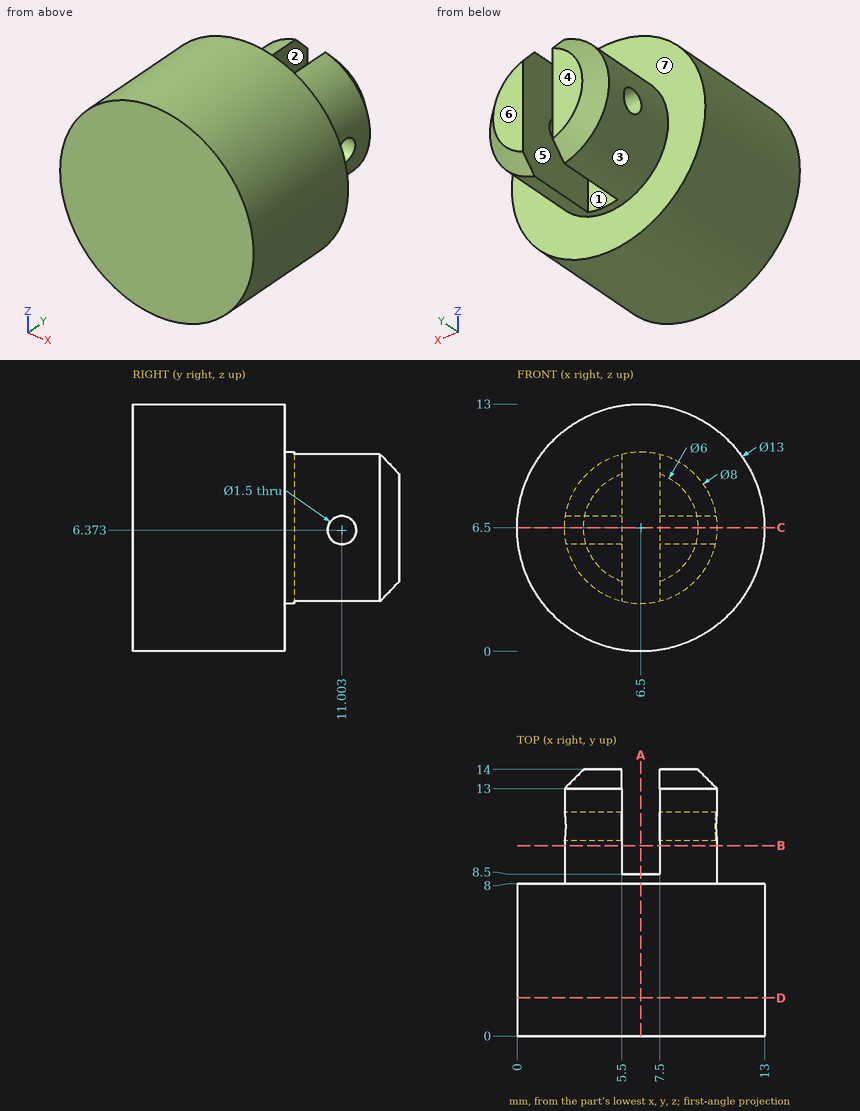
Here's the drawing with two shaded views (mm, measured from the low corner). I have some questions. A direction names the side the tool comes from. Round coordinates to 2 decimals unless told otherwise and drop trailing zeros. Order: outer loops, then holes, each group sorted by start corner. A loop starts at its lowest first (then second) coordinate and runs counter-clockwise, first axis right, second up. Notation, with made-up numbers: (86, 76.25) -> (100, 76.25) arc R17 cw to (100, 97.25) -> close; hole circle Ø5 at (68.25, 38.5). An arc over 180 degrees is marked (long way). Use a Markdown table: item, result. Add a question column.
(1) If we mould it in two halves opening along X, with no side actions, what happens to the marked faces 1, 2, 3 and 4? For each: released by +X, released by -X, zero draft, split by the parting line, or undercut.
(2) Suppose I cut it at D-D, the plane y = 2. Please give me the cut outline in (x, z).
(3) For pin 1 Ø1.2 at (y, z) = (11, 6.37) entering from -X; pin 2 Ø1.7 at (y, z) = (11, 6.37) entering from -X; pin 3 Ø4.5 at (y, z) = (10.5, 7) entering from +X; pin 4 Ø4 at (x, z) = (10.5, 3) entering from +Y (1 decimal), each with a flat end and sliding along its axis, tell me the tip position at first contact or that it passes through.
(4) Suppose I cut it at A-A, the plane x = 6.5. Please give me the cut outline in (y, z), and give its area (3 significant figures).
(5) Suppose I cut it at C-C, the plane z = 6.5. Please give me the cut outline in (x, y), and give its area (3 significant figures).
(6) Suppose I cut it at B-B, the plane y = 10. Please give me the cut outline in (x, z).
(7) I need wall thicknesses on line 1 along Y through (x, z) = (9.5, 12); line 2 along Y through (x, z) = (3.25, 7) (1 decimal); line 3 along X through (y, z) = (11, 9.75). Which ranges of each line are inside material? Lowest first, please.
(8) For the marked faces 5, 6 and 7, which set-ups out of +Z, -Z, +X, -X, +Y, -Y let a thin tool reach every point of the face, with its end or its side?
Verdict:
| question | item | result |
|---|---|---|
| 1 | face 1 | undercut |
| 1 | face 2 | undercut |
| 1 | face 3 | split by the parting line |
| 1 | face 4 | zero draft |
| 2 | outline | circle Ø13 at (6.5, 6.5) |
| 3 | pin 1 | through |
| 3 | pin 2 | x = 2.5 |
| 3 | pin 3 | x = 10.5 |
| 3 | pin 4 | y = 13.7 |
| 4 | outline | (0, 0) -> (8, 0) -> (8, 2.5) -> (8.5, 2.5) -> (8.5, 10.5) -> (8, 10.5) -> (8, 13) -> (0, 13) -> close |
| 4 | area | 108 mm2 |
| 5 | outline | (0, 0) -> (13, 0) -> (13, 8) -> (10.5, 8) -> (10.5, 10.26) -> (7.5, 10.26) -> (7.5, 8.5) -> (5.5, 8.5) -> (5.5, 10.26) -> (2.5, 10.26) -> (2.5, 8) -> (0, 8) -> close; (2.5, 11.74) -> (5.5, 11.74) -> (5.5, 14) -> (3.5, 14) -> (2.5, 13) -> close; (7.5, 11.74) -> (10.5, 11.74) -> (10.5, 13) -> (9.5, 14) -> (7.5, 14) -> close |
| 5 | area | 131 mm2 |
| 6 | outline | (5.5, 2.63) -> (5.5, 10.37) arc R4 ccw to start; (7.5, 2.63) arc R4 ccw to (7.5, 10.37) -> close |
| 7 | line 1 | 0 to 8 |
| 7 | line 2 | 0 to 10.6, 11.4 to 13.7 |
| 7 | line 3 | 4.17 to 5.5, 7.5 to 8.83 |
| 8 | face 5 | +Z, -Z, +Y |
| 8 | face 6 | +Z, -Z, +X, -X, +Y |
| 8 | face 7 | +Y |
